```python
from build123d import *

# Parameters (mm, degrees)
SKETCH1_W             = 40
SKETCH1_H             = 40
BOSS_EXTRUDE1_DEPTH   = 500
BOSS_EXTRUDE1_2_DEPTH = 500
BOSS_EXTRUDE1_3_DEPTH = 500
BOSS_EXTRUDE1_4_DEPTH = 500
SKETCH2_W             = 460
SKETCH2_H             = 300
SKETCH2_W_2           = 380
SKETCH2_H_2           = 220
BOSS_EXTRUDE2_DEPTH   = 30
BOSS_EXTRUDE4_REACH   = 694.676
SKETCH4_W             = 30
SKETCH4_H             = 30


with BuildPart() as part:
    # Sketch1 → Boss-Extrude1 (new body)
    with BuildSketch(Plane(origin=(0, 0, 0), x_dir=(1, 0, 0), z_dir=(0, 1, 0))):
        with Locations((-210, 130)):
            Rectangle(SKETCH1_W, SKETCH1_H)
    extrude(amount=BOSS_EXTRUDE1_DEPTH)



with BuildPart() as body_2:
    # Sketch1 → Boss-Extrude1 2 (new body)
    with BuildSketch(Plane(origin=(0, 0, 0), x_dir=(1, 0, 0), z_dir=(0, 1, 0))):
        with Locations((-210, -130)):
            Rectangle(SKETCH1_W, SKETCH1_H)
    extrude(amount=BOSS_EXTRUDE1_2_DEPTH)


with BuildPart() as body_3:
    # Sketch1 → Boss-Extrude1 3 (new body)
    with BuildSketch(Plane(origin=(0, 0, 0), x_dir=(1, 0, 0), z_dir=(0, 1, 0))):
        with Locations((210, -130)):
            Rectangle(SKETCH1_W, SKETCH1_H)
    extrude(amount=BOSS_EXTRUDE1_3_DEPTH)


with BuildPart() as body_4:
    # Sketch1 → Boss-Extrude1 4 (new body)
    with BuildSketch(Plane(origin=(0, 0, 0), x_dir=(1, 0, 0), z_dir=(0, 1, 0))):
        with Locations((210, 130)):
            Rectangle(SKETCH1_W, SKETCH1_H)
    extrude(amount=BOSS_EXTRUDE1_4_DEPTH)


with BuildPart() as part_1:
    add(part.part)

    add(body_2.part)  # Boss-Extrude2 merges body 2

    add(body_3.part)  # Boss-Extrude2 merges body 3

    add(body_4.part)  # Boss-Extrude2 merges body 4
    # Sketch2 → Boss-Extrude2 (add)
    with BuildSketch(Plane(origin=(0, 500, 0), x_dir=(1, 0, 0), z_dir=(0, 1, 0))):
        Rectangle(SKETCH2_W, SKETCH2_H)
        Rectangle(SKETCH2_W_2, SKETCH2_H_2, mode=Mode.SUBTRACT)
    extrude(amount=BOSS_EXTRUDE2_DEPTH)

    # Sketch4 → Boss-Extrude4 (add, up to next)
    with BuildSketch(Plane(origin=(-190, 0, 0), x_dir=(0, 0, -1), z_dir=(1, 0, 0)), mode=Mode.PRIVATE) as boss_extrude4_sk1:
        with Locations((-65, 515)):
            Rectangle(SKETCH4_W, SKETCH4_H)
    boss_extrude4_tool1 = extrude(boss_extrude4_sk1.sketch, amount=BOSS_EXTRUDE4_REACH, mode=Mode.PRIVATE) - part_1.part
    # Sketch4 → Boss-Extrude4 (add, up to next)
    with BuildSketch(Plane(origin=(-190, 0, 0), x_dir=(0, 0, -1), z_dir=(1, 0, 0)), mode=Mode.PRIVATE) as boss_extrude4_sk2:
        with Locations((0, 515)):
            Rectangle(SKETCH4_W, SKETCH4_H)
    boss_extrude4_tool2 = extrude(boss_extrude4_sk2.sketch, amount=BOSS_EXTRUDE4_REACH, mode=Mode.PRIVATE) - part_1.part
    # Sketch4 → Boss-Extrude4 (add, up to next)
    with BuildSketch(Plane(origin=(-190, 0, 0), x_dir=(0, 0, -1), z_dir=(1, 0, 0)), mode=Mode.PRIVATE) as boss_extrude4_sk3:
        with Locations((65, 515)):
            Rectangle(SKETCH4_W, SKETCH4_H)
    boss_extrude4_tool3 = extrude(boss_extrude4_sk3.sketch, amount=BOSS_EXTRUDE4_REACH, mode=Mode.PRIVATE) - part_1.part
    add(boss_extrude4_tool1.solids().sort_by_distance((-190, 515, 65))[0])
    add(boss_extrude4_tool2.solids().sort_by_distance((-190, 515, 0))[0])
    add(boss_extrude4_tool3.solids().sort_by_distance((-190, 515, -65))[0])


solid = part_1.part
```
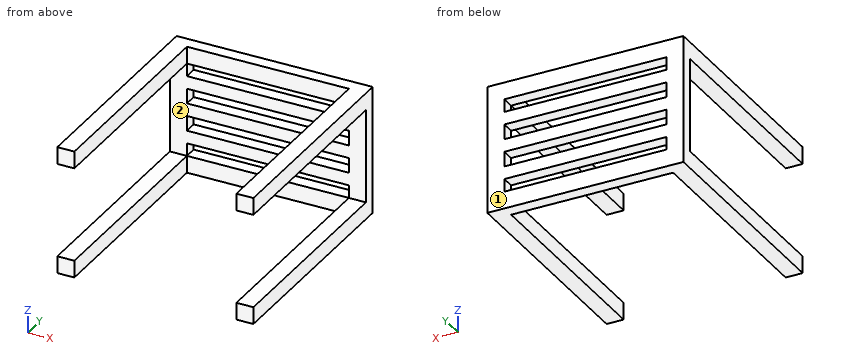
Source: CAD feature listing. Evaluate the final solid. Frame: model axes, mm. Face numbers are marked on the shaded views. Give positions to 0.01 mm unless a question says otherwise; leave off trailing zeros. Write each loop counter-clockwise with the first axis right and the second up, starting at its lowest first coordinate (ties: lowest second). Pieces come first, ordered by that corner, then holes. Notation, with made-up numbers: (-23, 39) - (33, 39) arc R16 ccw to (33, 49) - close; hole circle Ø5 at (80, -39.5). An arc over 180 degrees is marked (long way). One line per item, written item: value. Start each with the question number.
Q1. Section query C-C, the plane x = 148. Return the cut outline in (y, z), then the cut area to 3 significant figures.
Q2. Section query B-B, the plane z = -95. Return the cut outline in (x, y), then the cut area to 3 significant figures.
Q3. Section query D-D, the plane x = 202.5. Return the cut outline in (y, z), then the cut area to 3 significant figures.
Q4. Draft query along Z for the marked faces 1 and 2. Return one class per face: +Z half, -Z half, draft (parallel to the pull), parting line (faces both ways), or undercut.
Q5. Section query A-A, the plane y = 259.5. Return the cut outline in (x, z).
Q6. First-contact query: pin 1 Ø5 at (x, z) = (50, 84) entering from +Y. Flat tip, straight axial feed; report the tip coordinate or a pass-through.
Q7. Material intervals for probe 1 along Z at (x, y) = (198.5, 232.5); probe 2 along X at (y, z) = (126, -134); probe 3 along Y at (x, z) = (115, 131.5), sorted ascending. Write a range as from..to.
Answer:
1. outline: (500, -150) - (530, -150) - (530, -110) - (500, -110) - close; (500, -80) - (530, -80) - (530, -50) - (500, -50) - close; (500, -15) - (530, -15) - (530, 15) - (500, 15) - close; (500, 50) - (530, 50) - (530, 80) - (500, 80) - close; (500, 110) - (530, 110) - (530, 150) - (500, 150) - close
1. area: 5,100 mm2
2. outline: (-230, 500) - (-190, 500) - (-190, 530) - (-230, 530) - close; (190, 500) - (230, 500) - (230, 530) - (190, 530) - close
2. area: 2,400 mm2
3. outline: (0, -150) - (530, -150) - (530, 150) - (0, 150) - (0, 110) - (500, 110) - (500, -110) - (0, -110) - close
3. area: 49,000 mm2
4. face 1: draft
4. face 2: undercut
5. outline: (-230, -150) - (-190, -150) - (-190, -110) - (-230, -110) - close; (-230, 110) - (-190, 110) - (-190, 150) - (-230, 150) - close; (190, -150) - (230, -150) - (230, -110) - (190, -110) - close; (190, 110) - (230, 110) - (230, 150) - (190, 150) - close
6. pin 1: passes through
7. probe 1: z = -150..-110, 110..150
7. probe 2: x = -230..-190, 190..230
7. probe 3: y = 500..530
